Job drawing, mm, ordinate dimensions from the low corner. One solid piece. A direction names the side the tool comes from. Coordinates: 2 decimals unless noted, no trailing zeros. Write each loop counter-clockwise with the first axis right and the second up, starting at its lowest first coordinate (ties: lowest second). Pieces come first, ordered by that corner, then holes. Notation, with made-up numbers: (5, 0.5) - (22, 0.5) arc R16 cw to (22, 8.5) - close; hole circle Ø8 at (53, 60.25). An arc over 180 degrees is marked (long way). Use a Markdown table: item, result.
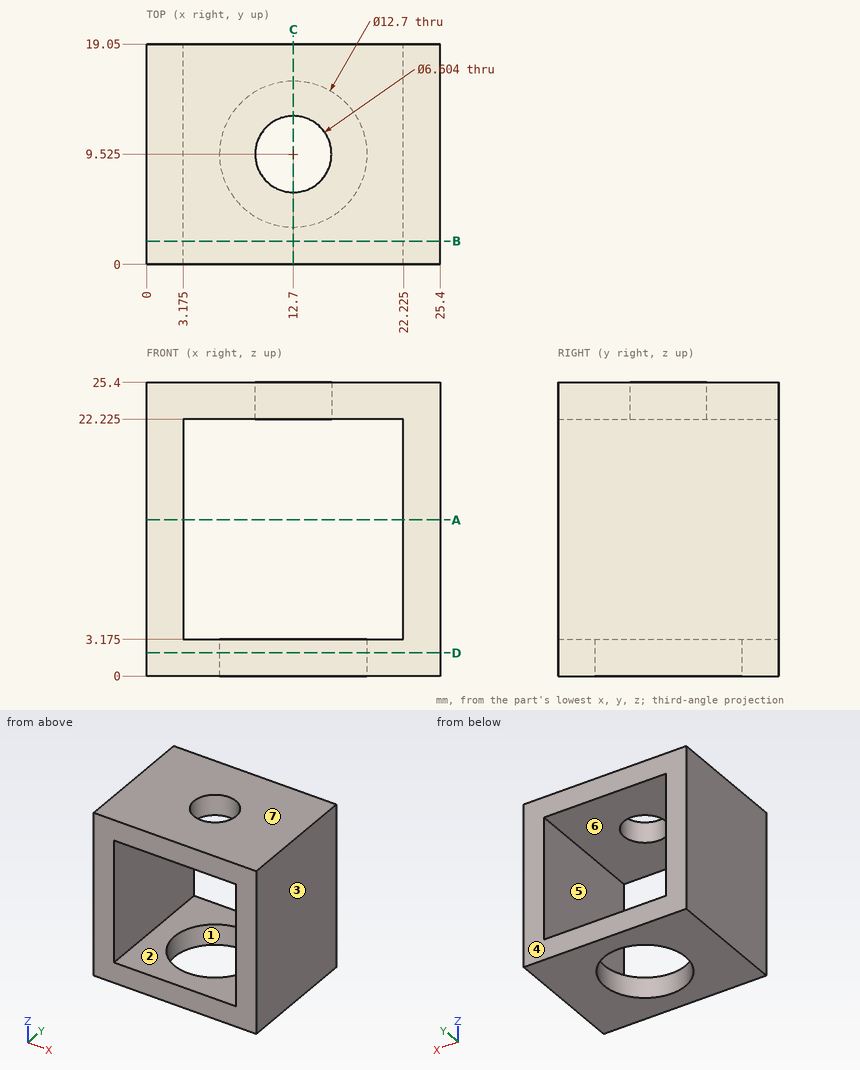
Item 1: Band-saw the part on C-C, the plane x = 12.7. Give the cut face in (y, z) (3 decimals).
From the geometry:
| item | result |
|---|---|
| outline | (0, 0) - (3.175, 0) - (3.175, 3.175) - (0, 3.175) - close; (0, 22.225) - (6.223, 22.225) - (6.223, 25.4) - (0, 25.4) - close; (12.827, 22.225) - (19.05, 22.225) - (19.05, 25.4) - (12.827, 25.4) - close; (15.875, 0) - (19.05, 0) - (19.05, 3.175) - (15.875, 3.175) - close |
Item 2: Which spindle directions (+Z, -Z, +X, -X, +Y, -Y) get a long thin tool onto all of the face, cutting with end or side? Do the marked faces 1, 2 and 3. Say none if no direction does.
From the geometry:
| item | result |
|---|---|
| face 1 | -Z |
| face 2 | +Y, -Y |
| face 3 | +Z, -Z, +X, +Y, -Y |
Item 3: Two-plate mould, pull along Z, no slides. Class the marked faces 4, 5, 6 and 7: pulls with the +Z half, pulls with the -Z half, needs draft (parallel to the pull), parting line crosses it, or undercut.
From the geometry:
| item | result |
|---|---|
| face 4 | needs draft |
| face 5 | undercut |
| face 6 | undercut |
| face 7 | pulls with the +Z half |
Item 4: Band-saw the part on A-A, the plane z = 13.5. Give the cut face in (x, y) (3 decimals), then the cut area to 3 significant figures.
From the geometry:
| item | result |
|---|---|
| outline | (0, 0) - (3.175, 0) - (3.175, 19.05) - (0, 19.05) - close; (22.225, 0) - (25.4, 0) - (25.4, 19.05) - (22.225, 19.05) - close |
| area | 121 mm^2 |
Item 5: Drill centre lines: probe 1 along X at (y, z) = (8.75, 21.75) (3 decimals); probe 2 along Y at (x, z) = (12.7, 24.4). Where is each one in solid material? Low to high.
From the geometry:
| item | result |
|---|---|
| probe 1 | 0 to 3.175, 22.225 to 25.4 |
| probe 2 | 0 to 6.22, 12.83 to 19.05 |
Item 6: Band-saw the part on B-B, the plane y = 2. Give the cut face in (x, z) (3 decimals).
From the geometry:
| item | result |
|---|---|
| outline | (0, 0) - (25.4, 0) - (25.4, 25.4) - (0, 25.4) - close; hole (3.175, 3.175) - (22.225, 3.175) - (22.225, 22.225) - (3.175, 22.225) - close |
Item 7: Band-saw the part on D-D, the plane z = 2. Give the cut face in (x, y) (3 decimals).
From the geometry:
| item | result |
|---|---|
| outline | (0, 0) - (25.4, 0) - (25.4, 19.05) - (0, 19.05) - close; hole circle Ø12.7 at (12.7, 9.525) |
Item 8: Drop a flat-ended pin along its axis: P1, Ø1.5, axis at x = 19, z = 4.5, coming from the +Y side. Give the stop position or say it passes through.
From the geometry:
| item | result |
|---|---|
| P1 | through |
